Here's the drawing with two shaded views (mm, measured from the low corner). I have some questions. A direction names the side the tool comes from. Round coordinates to 2 decimals unless told otherwise and drop trailing zeros. Loops run counter-clockwise (first coordinate to the right, second up) from the corner with the lowest first, then second, coordinate; pieces in that order, holes last.
(1) I want a section at C-C on z = 150.5. Write out the boundary of the cut face in (x, y), plus the area to 3 significant figures.
(2) Which directions (+Z, -Z, +X, -X, +Y, -Y) give clear straight access to the entire face, cutting with the end or side of a thin tool? Please do the marked faces 1, 2 and 3.
(3) Thinking about a two-plate mould opening in X: for the marked faces 4 and 5, which applies, released by +X, released by -X, zero draft, split by the parting line, or undercut?
(4) I want a section at B-B on x = 70. Write out the boundary of the cut face in (y, z).
(5) Will these pins go through, and if not, where does the flat tip stop? pin 1 Ø5 at (x, y) = (31, 120) entering from -Z; pin 2 Ø10 at (x, z) = (118.5, 91) entering from +Y; pin 3 Ø5 at (x, z) = (113, 147.5) entering from +Y (1 decimal).
(6) I want a section at D-D on x = 26. Write out the boundary of the cut face in (y, z), plus the area to 3 significant figures.
(7) I want a section at A-A on y = 70. Write out the boundary of the cut face in (x, z).
(8) If I drill on line 1 along Z through (x, y) = (50, 26); line 2 along Z through (x, y) = (73, 45.5); line 3 along Y through (x, z) = (72, 185), over which ranges is the centre line in solid material (lowest first)?
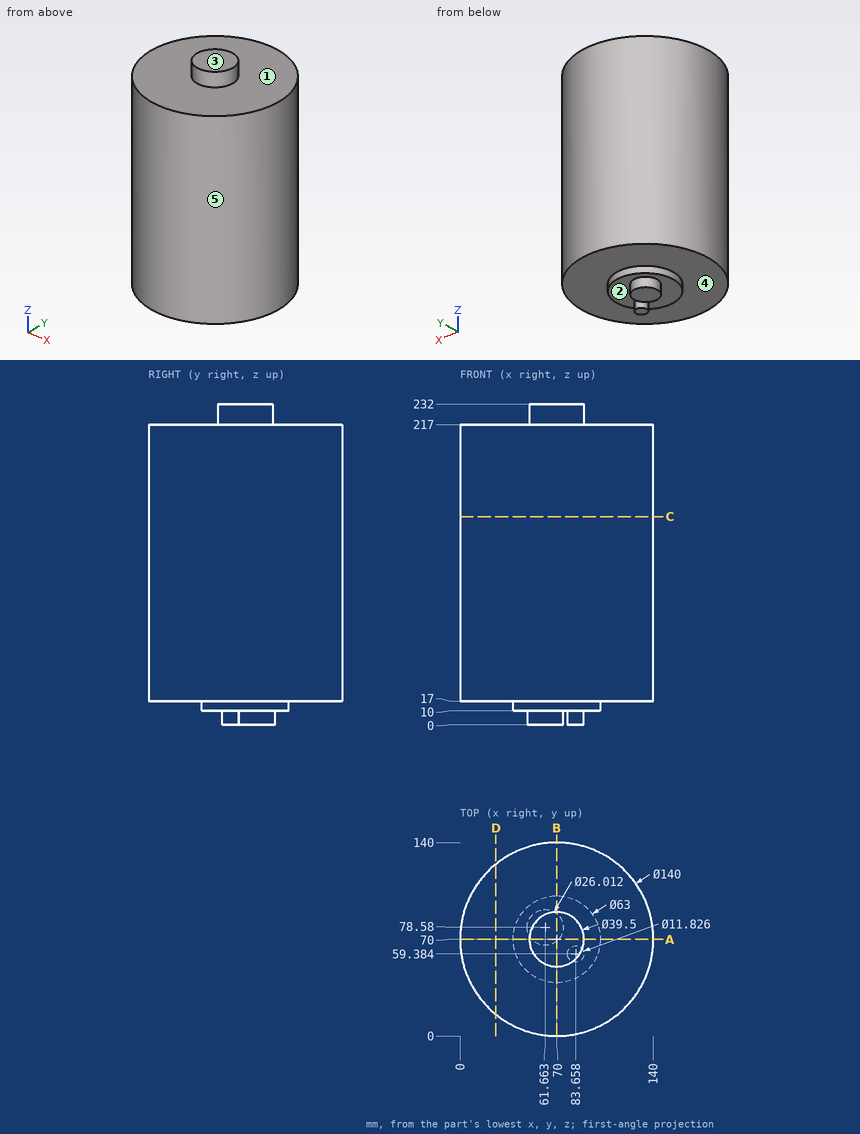
Filled sheet:
1. outline: circle Ø140 at (70, 70)
1. area: 15,400 mm2
2. face 1: +Z
2. face 2: -Z
2. face 3: +Z, +X, -X, +Y, -Y
3. face 4: zero draft
3. face 5: split by the parting line
4. outline: (0, 17) - (38.5, 17) - (38.5, 10) - (68.6, 10) - (68.6, 0) - (88.56, 0) - (88.56, 10) - (101.5, 10) - (101.5, 17) - (140, 17) - (140, 217) - (89.75, 217) - (89.75, 232) - (50.25, 232) - (50.25, 217) - (0, 217) - close
5. pin 1: stops at z = 17
5. pin 2: stops at y = 124.84
5. pin 3: stops at y = 127.1
6. outline: (15.56, 17) - (124.44, 17) - (124.44, 217) - (15.56, 217) - close
6. area: 21,800 mm2
7. outline: (0, 17) - (38.5, 17) - (38.5, 10) - (51.89, 10) - (51.89, 0) - (71.44, 0) - (71.44, 10) - (101.5, 10) - (101.5, 17) - (140, 17) - (140, 217) - (89.75, 217) - (89.75, 232) - (50.25, 232) - (50.25, 217) - (0, 217) - close
8. line 1: z = 17 to 217
8. line 2: z = 10 to 217
8. line 3: y = 0.03 to 139.97
